from build123d import *

# Parameters (mm, degrees)
F0_W     = 20
F0_H     = 22
F1_DEPTH = 2
F2_R     = 9.25
F4_DEPTH = 2
F3_W     = 20
F3_H     = 18
F5_DEPTH = 2
F6_W     = 20
F6_H     = 0.75
F7_DEPTH = 2
F8_R     = 125
F9_DEPTH = 2
F10_R    = 1


with BuildPart() as f1:
    # F0 (on Top) → F1 (new body)
    with BuildSketch(Plane.XY):
        Rectangle(F0_W, F0_H)
    extrude(amount=F1_DEPTH)

    # F2 (on face) → F4 (join)
    with BuildSketch(Plane.XY.offset(2)):
        with Locations((0, -1.25)):
            Circle(F2_R)
    extrude(amount=F4_DEPTH)

    # F3 (on face) → F5 (cut)
    with BuildSketch(Plane.XY.offset(2)):
        with Locations((0, -3.5)):
            Rectangle(F3_W, F3_H)
    extrude(amount=F5_DEPTH, mode=Mode.SUBTRACT)

    # F6 (on face) → F7 (join)
    with BuildSketch(Plane.XY.offset(2)):
        with Locations((0, 10.625)):
            Rectangle(F6_W, F6_H)
    extrude(amount=F7_DEPTH)

    # F8 (on Top) → F9 (cut)
    with BuildSketch(Plane.XY):
        with Locations((0, -132.75)):
            Circle(F8_R)
    extrude(amount=F9_DEPTH, mode=Mode.SUBTRACT)

    # F10
    f10_edges = [f1.edges().sort_by_distance(p)[0] for p in [
        (10, -8.150642, 1),
        (-10, -8.150642, 1),
        (10, 11, 2),
        (-10, 11, 2),
        (0, 11, 0),
        (-10, 1.424679, 0),
        (0, -7.75, 0),
        (10, 1.424679, 0),
    ]]
    fillet(f10_edges, radius=F10_R)


solid = f1.part
Can you work these out from the model? Positions are in its coordinate system, mm. A direction names the side the tool comes from. Round coordinates to 2 decimals unless told otherwise and drop trailing zeros. Write each loop counter-clockwise with the first axis right and the second up, starting at its lowest first coordinate (ties: lowest second). Pieces come first, ordered by that corner, then holes. Notation, with made-up numbers: (28, 44.25) -> (56, 44.25) arc R34 ccw to (56, 75.25) -> close; hole circle Ø8 at (65.5, 8.5). An arc over 180 degrees is marked (long way). One line per question, with ' | ' between items. Start each with the question number.
1) Suppose I cut it at B-B on y = 2.5. Write out the boundary of the cut face in (x, z), then the cut area to 3 significant figures.
2) If we mould it in two halves opening along X, with no side actions, what happens to faces 1 (the cylindrical face through (9.699, 1.584, 0.285)), 2 (the cylindrical face through (-9.6, 10.8, 2.5)), 3 (the cylindrical face through (0.13, -7.75, 1.49)), 4 (the flat face through (0, 5.5, 3))? For each: released by +X, released by -X, zero draft, split by the parting line, or undercut.
3) On a 3-axis mill with a long thin cutter (end or side, diameter ignored), from which of +Z, -Z, +X, -X, +Y, -Y can I reach the whole of each face in a straight line? I mean faces 5 (the flat face through (0, 6, 4)), 6 (the cylindrical face through (0, 8, 3)), 7 (the flat face through (0, 10.25, 3)). Say none if no direction works.
4) Suppose I cut it at A-A on z = 2.35. Write out the boundary of the cut face in (x, y).
5) I need wall thicknesses on line 1 (Y direction, x = -0.25, z = 3.75); line 2 (Z direction, x = -1.25, y = 5); line 3 (Y direction, x = 7, z = 3). Which ranges of each line are inside material? Lowest first, please. Write a range as [from, to].
6) I'm going to push flat-ended pins straight in: P1, Ø1, axis at x = 3.5, z = 3.5, coming from the -Y side; P2, Ø1.5, axis at x = -2.5, z = 0.5, coming from the -Y side. Where does each tip first touch, or does it pass through?
Return value:
1) outline: (-10, 1) arc R1 ccw to (-9, 0) -> (9, 0) arc R1 ccw to (10, 1) -> (10, 2) -> (-10, 2) -> close | area: 39.6 mm2
2) face 1: released by +X | face 2: released by -X | face 3: undercut | face 4: zero draft
3) face 5: +Z, +X, -X, +Y, -Y | face 6: +Z | face 7: +Z, +X, -X
4) outline: (-9.97, 10.25) -> (9.97, 10.25) arc R1 ccw to (9, 11) -> (-9, 11) arc R1 ccw to start; (-6.32, 5.5) -> (6.32, 5.5) arc R9.25 ccw to start
5) line 1: y = [5.5, 8], [10.25, 11] | line 2: z = [0, 2] | line 3: y = [10.25, 11]
6) P1: stops at y = 5.5 | P2: stops at y = -7.79
